Study the drawing (mm; zero at the part's minimum x, y, z) and answer. A direction names the side the tool comes from. Coordinates: 2 decimals unless noted, no trailing zeros. Loops run counter-clockwise (first coordinate to the right, second up) from the corner with the lowest first, then second, coordinate; pieces in that order, holes last.
Q1. Section B-B (z = 7.5) is taken. Give the vertices of the cut face in (x, y).
Q2. A straight line is drawn through the part: line 1 (Y direction, x = 14.5, z = 9.5). Find the intervals that lie inside material, in ascending order.
Q3. Section D-D (y = 16.5) is taken. Give the vertices of the cut face in (x, z).
Q4. Flat-ended cylindrical pins translate along their axes: P1, Ø3, axis at x = 14, y = 7, coming from the +Z side; P2, Ø3, axis at x = 13, z = 5.5, coming from the +Y side; P3, Ø4, axis at y = 26.5, z = 12, coming from the +X side. Find the tip coordinate at first contact, or state that the pin passes through.
Q5. Section C-C (x = 14.5) is taken. Give the vertices of the cut face in (y, z).
Q6. Section A-A (y = 4.5) is taken. Give the vertices of the cut face in (x, z), then the cut area to 3 significant figures.
Q7. Which of the six approach directions +Z, -Z, +X, -X, +Y, -Y give full straight-line access (tool end or side, diameter ignored) to the marked faces 1, 2 and 3?
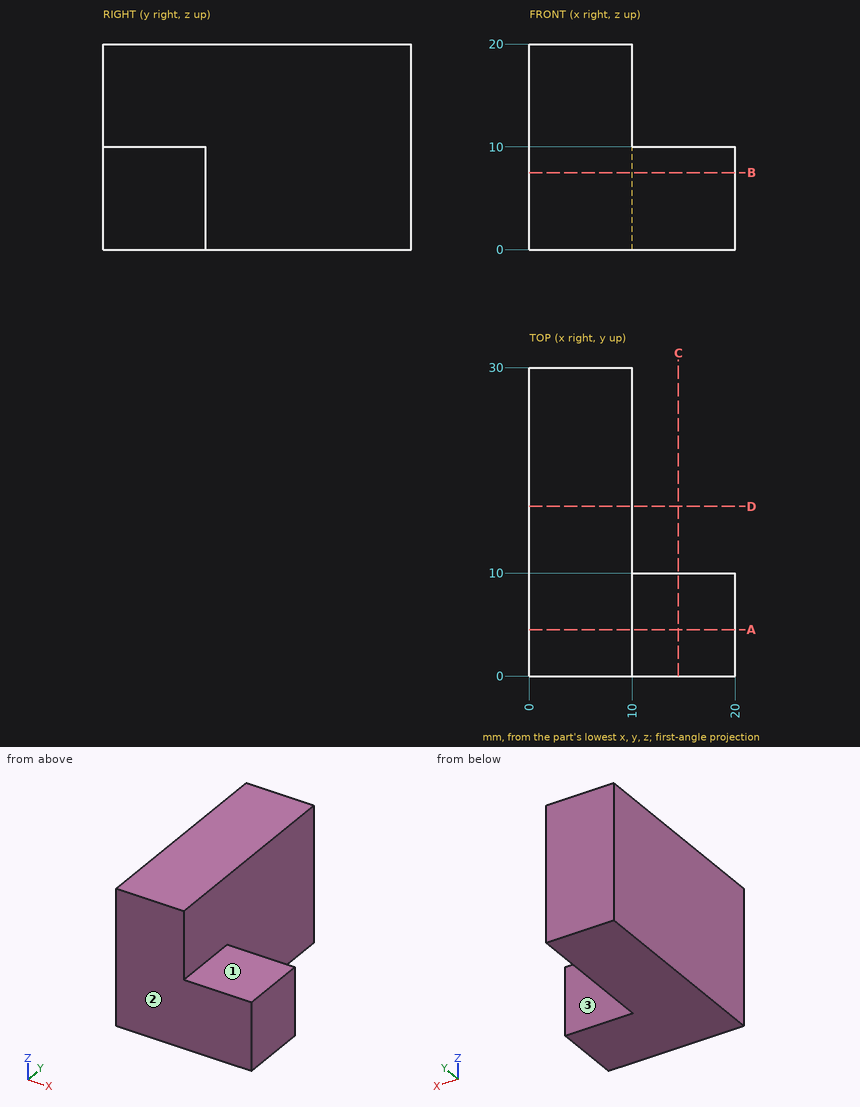
Numbers:
1. outline: (0, 0) - (20, 0) - (20, 10) - (10, 10) - (10, 30) - (0, 30) - close
2. line 1: y = 0 to 10
3. outline: (0, 0) - (10, 0) - (10, 20) - (0, 20) - close
4. P1: stops at z = 10
4. P2: stops at y = 10
4. P3: stops at x = 10
5. outline: (0, 0) - (10, 0) - (10, 10) - (0, 10) - close
6. outline: (0, 0) - (20, 0) - (20, 10) - (10, 10) - (10, 20) - (0, 20) - close
6. area: 300 mm2
7. face 1: +Z, +X, +Y, -Y
7. face 2: +Z, -Z, +X, -X, -Y
7. face 3: +Z, -Z, +X, +Y
